from build123d import *

# Parameters (mm, degrees)
SALIENTE_EXTRUIR1_DEPTH = 20
REDONDEO1_RADIUS        = 0.5
REDONDEO1_LENGTH        = 20
REDONDEO3_R             = 1
REDONDEO4_R             = 1
CROQUIS6_W              = 0.519230147
CROQUIS6_H              = 1.134138633
CORTAR_EXTRUIR2_DEPTH   = 31
CROQUIS7_W              = 1.5
CROQUIS7_H              = 20
SALIENTE_EXTRUIR2_DEPTH = 2
REDONDEO5_RADIUS        = 0.75
REDONDEO5_LENGTH        = 20


with BuildPart() as part:
    # Croquis3 → Saliente-Extruir1 (new body)
    with BuildSketch(Plane(origin=(0, 0, 0), x_dir=(1, 0, 0), z_dir=(0, 1, 0))):
        Polygon((-2.726281257, 0), (-4.017413973, 0), (-4.017413973, -3.1), (9.282586027, -3.1), (9.282586027, 4), (7.282586027, 4), (7.282586027, 3), (8.282586027, 3), (8.282586027, -2.1), (-3.017413973, -2.1), (-3.017413973, -1), (-2.726281257, -1), align=None)
    extrude(amount=SALIENTE_EXTRUIR1_DEPTH)

    # Redondeo1: full round fillet: the end face becomes a half cylinder, R = half its width
    redondeo1_face = Plane((7.282586027, 10, -3.5), x_dir=(0, 1, 0), z_dir=(-1, 0, 0))  # on the end face: x along it, z out of the body
    redondeo1_slab = redondeo1_face.offset(-REDONDEO1_RADIUS / 2) * Box(REDONDEO1_LENGTH, 2 * REDONDEO1_RADIUS, REDONDEO1_RADIUS, mode=Mode.PRIVATE)  # the body's end, R deep
    redondeo1_round = Plane((7.782586027, 10, -3.5), x_dir=(-1, 0, 0), z_dir=(0, 1, 0)) * Cylinder(REDONDEO1_RADIUS, REDONDEO1_LENGTH, mode=Mode.PRIVATE)  # its axis R under the face
    add(redondeo1_slab - redondeo1_round, mode=Mode.SUBTRACT)

    # Redondeo3
    redondeo3_edges = [part.edges().sort_by_distance(p)[0] for p in [
        (-4.017413973, 10, 3.1),
    ]]
    fillet(redondeo3_edges, radius=REDONDEO3_R)

    # Redondeo4
    redondeo4_edges = [part.edges().sort_by_distance(p)[0] for p in [
        (9.282586027, 10, 3.1),
    ]]
    fillet(redondeo4_edges, radius=REDONDEO4_R)

    # Croquis6 → Cortar-Extruir2 (cut)
    with BuildSketch(Plane(origin=(0, 20, 0), x_dir=(1, 0, 0), z_dir=(0, 1, 0))):
        with Locations((-2.7577989, -0.432930683)):
            Rectangle(CROQUIS6_W, CROQUIS6_H)
    extrude(amount=-CORTAR_EXTRUIR2_DEPTH, mode=Mode.SUBTRACT)

    # Croquis7 → Saliente-Extruir2 (add)
    with BuildSketch(Plane(origin=(9.282586027, 0, 0), x_dir=(0, 0, -1), z_dir=(1, 0, 0))):
        with Locations((1.7, 10)):
            Rectangle(CROQUIS7_W, CROQUIS7_H)
    extrude(amount=SALIENTE_EXTRUIR2_DEPTH)

    # Redondeo5: full round fillet: the end face becomes a half cylinder, R = half its width
    redondeo5_face = Plane((11.282586027, 10, -1.7), x_dir=(0, -1, 0), z_dir=(1, 0, 0))  # on the end face: x along it, z out of the body
    redondeo5_slab = redondeo5_face.offset(-REDONDEO5_RADIUS / 2) * Box(REDONDEO5_LENGTH, 2 * REDONDEO5_RADIUS, REDONDEO5_RADIUS, mode=Mode.PRIVATE)  # the body's end, R deep
    redondeo5_round = Plane((10.532586027, 10, -1.7), x_dir=(1, 0, 0), z_dir=(0, -1, 0)) * Cylinder(REDONDEO5_RADIUS, REDONDEO5_LENGTH, mode=Mode.PRIVATE)  # its axis R under the face
    add(redondeo5_slab - redondeo5_round, mode=Mode.SUBTRACT)


solid = part.part
Model file for the job. Use its own axes, mm. A direction names the side the tool comes from. Round coordinates to 2 decimals unless told otherwise and drop trailing zeros. Loops run counter-clockwise (first coordinate to the right, second up) from the corner with the lowest first, then second, coordinate; pieces in that order, holes last. Notation, with made-up numbers: M 79.25,60 L 97.25,60 A19 ccw 97.25,83 Z; hole C 74,-1 d4. An arc over 180 degrees is marked long. One line per question, with ' | ' between items.
1) Band-saw the part on A-A (z = 0.75). Give the cut face in (x, y).
Solved:
outline: M -4.02,0 L -3.02,0 L -3.02,20 L -4.02,20 Z; M 8.28,0 L 9.28,0 L 9.28,20 L 8.28,20 Z
2) Mould opens along Z. For faces 1 (the flat face through (-3.5, 9.9, 0)), 2 (the flat face through (8.283, 10, 0)), 3 (the flat face through (9.283, 10, -3)) say: +Z half, -Z half, draft (parallel to the pull), parting line (faces both ways), or undercut.
Solved:
face 1: -Z half | face 2: undercut | face 3: draft
3) Flat gauge pins, fed straight in: pin 1 (1 mm diameter, centred on x = 9.5, y = 8, fed in from +Z); pin 2 (4 mm diameter, centred on y = 11, z = -1.5, fed in from -X); pin 3 (1 mm diameter, centred on y = 2.5, z = -1.5, fed in from -X); pin 4 (1.5 mm diameter, centred on y = 11, z = -2.5, fed in from -X). Where does each tip first touch, or does it go through?
Solved:
pin 1: stops at z = 2.8 | pin 2: stops at x = -4.02 | pin 3: stops at x = 8.28 | pin 4: stops at x = 7.35
4) Band-saw the part on C-C (x = 9.5). Give the cut face in (y, z), then the cut area to 3 significant figures.
Solved:
outline: M 0,-2.45 L 20,-2.45 L 20,-0.95 L 0,-0.95 Z | area: 30.0 mm²
5) Drill centre lines: line 1 along X through (y, z) = (9.5, 1.25); line 2 along Z through (x, y) = (6.25, 13.75); line 3 along X through (y, z) = (17.75, -1.75). Where is each one in solid material? Low to high.
Solved:
line 1: x = -4.02 to -3.02, 8.28 to 9.28 | line 2: z = 2.1 to 3.1 | line 3: x = 8.28 to 11.28
6) 3-axis set-ups, long thin cutter, end or side, ignore diameter. For faces 4 (the flat face through (-3.017, 10, 1)), 5 (the flat face through (9.283, 10, 1)), 6 (the flat face through (10, 10, -2.45)): which of +Z, -Z, +X, -X, +Y, -Y reach the whole face in a straight line?
Solved:
face 4: -Z, +Y, -Y | face 5: +Z, +X, +Y, -Y | face 6: -Z, +X, +Y, -Y
7) Band-saw the part on B-B (y = 7.25). Give the cut face in (x, z).
Solved:
outline: M -4.02,0 L -3.02,0 L -3.02,2.1 L 8.28,2.1 L 8.28,-3 L 7.78,-3 A0.5 ccw 7.78,-4 L 9.28,-4 L 9.28,-2.45 L 10.53,-2.45 A0.75 ccw 10.53,-0.95 L 9.28,-0.95 L 9.28,2.1 A1 ccw 8.28,3.1 L -3.02,3.1 A1 ccw -4.02,2.1 Z
8) Band-saw the part on D-D (z = -1.7). Give the cut face in (x, y), then the cut area to 3 significant figures.
Solved:
outline: M 8.28,0 L 11.28,0 L 11.28,20 L 8.28,20 Z | area: 60.0 mm²
